Input: part model. Units: mm. Frame: model coordinates. A direction names the side the tool comes from. Give positions to 0.01 mm unless a question says otherwise; leave off trailing zeros. Loops run counter-clockwise (first coordinate to the right, second up) from the corner with the lowest first, then second, coordinate; pieces in that order, holes last. Notation, with made-up numbers: (-16, 36) -> (16, 36) arc R25 ccw to (16, 57) -> close; hole circle Ø3 at (87.25, -6). An arc over 180 degrees is marked (long way). Answer as a JSON object with one key per item and string values.
```python
from build123d import *

# Parameters (mm, degrees)
F0_R     = 12.5
F0_R_2   = 9.5
F0_R_3   = 3.5
F1_DEPTH = 20
F2_DEPTH = 5
F3_R     = 1.5
F4_SIZE  = 0.99999
F5_SIZE  = 1


# Not quite as in the source:
# - a fillet or chamfer is up to 0.001 mm smaller than in the source, because OpenCascade refuses the exact size


with BuildPart() as f1:
    # F0 (on Top) → F1 (new body)
    with BuildSketch(Plane.XY):
        with BuildLine():
            Line((50, 27.5), (-50, 27.5))
            ThreePointArc((-50, 27.5), (-53.5355339059, 26.0355339059), (-55, 22.5))
            Line((-55, 22.5), (-55, -22.5))
            ThreePointArc((-55, -22.5), (-53.5355339059, -26.0355339059), (-50, -27.5))
            Line((-50, -27.5), (50, -27.5))
            ThreePointArc((50, -27.5), (53.5355339059, -26.0355339059), (55, -22.5))
            Line((55, -22.5), (55, 22.5))
            ThreePointArc((55, 22.5), (53.5355339059, 26.0355339059), (50, 27.5))
        make_face()
        with Locations((-37.5, -12)):
            Circle(F0_R, mode=Mode.SUBTRACT)
        with BuildLine():
            ThreePointArc((0, -12), (-12.5, -24.5), (-25, -12))
            ThreePointArc((-25, -12), (-12.5, 0.5), (0, -12))
        make_face(mode=Mode.SUBTRACT)
        with BuildLine():
            ThreePointArc((25, -12), (12.5, -24.5), (0, -12))
            ThreePointArc((0, -12), (12.5, 0.5), (25, -12))
        make_face(mode=Mode.SUBTRACT)
        with BuildLine():
            ThreePointArc((50, -12), (37.5, -24.5), (25, -12))
            ThreePointArc((25, -12), (37.5, 0.5), (50, -12))
        make_face(mode=Mode.SUBTRACT)
        with Locations((-43, 15)):
            Circle(F0_R_2, mode=Mode.SUBTRACT)
        with Locations((-21.5, 15)):
            Circle(F0_R_2, mode=Mode.SUBTRACT)
        with Locations((0, 15)):
            Circle(F0_R_2, mode=Mode.SUBTRACT)
        with Locations((21.5, 15)):
            Circle(F0_R_2, mode=Mode.SUBTRACT)
        with Locations((43, 15)):
            Circle(F0_R_2, mode=Mode.SUBTRACT)
        with BuildLine():
            ThreePointArc((0, -12), (-12.5, 0.5), (-25, -12))
            ThreePointArc((-25, -12), (-12.5, -24.5), (0, -12))
        make_face()
        with Locations((-12.5, -12)):
            Circle(F0_R_3, mode=Mode.SUBTRACT)
        with Locations((-37.5, -12)):
            Circle(F0_R)
        with Locations((-37.5, -12)):
            Circle(F0_R_3, mode=Mode.SUBTRACT)
        with BuildLine():
            ThreePointArc((25, -12), (12.5, 0.5), (0, -12))
            ThreePointArc((0, -12), (12.5, -24.5), (25, -12))
        make_face()
        with Locations((12.5, -12)):
            Circle(F0_R_3, mode=Mode.SUBTRACT)
        with BuildLine():
            ThreePointArc((50, -12), (37.5, 0.5), (25, -12))
            ThreePointArc((25, -12), (37.5, -24.5), (50, -12))
        make_face()
        with Locations((37.5, -12)):
            Circle(F0_R_3, mode=Mode.SUBTRACT)
    extrude(amount=F1_DEPTH)

    # F0 (on Top) → F2 (join)
    with BuildSketch(Plane.XY):
        with Locations((-43, 15)):
            Circle(F0_R_2)
        with Locations((-21.5, 15)):
            Circle(F0_R_2)
        with Locations((0, 15)):
            Circle(F0_R_2)
        with Locations((21.5, 15)):
            Circle(F0_R_2)
        with Locations((43, 15)):
            Circle(F0_R_2)
    extrude(amount=F2_DEPTH)

    # F3
    f3_edges = [f1.edges().sort_by_distance(p)[0] for p in [
        (0, -27.5, 20),
    ]]
    fillet(f3_edges, radius=F3_R)

    # F4 (size 1 in the source; OpenCascade refuses exactly that, so slightly less here)
    f4_edges = [f1.edges().sort_by_distance(p)[0] for p in [
        (-52.5, 15, 20),
        (-31, 15, 20),
        (-9.5, 15, 20),
        (12, 15, 20),
        (33.5, 15, 20),
    ]]
    chamfer(f4_edges, length=F4_SIZE)

    # F5
    f5_edges = [f1.edges().sort_by_distance(p)[0] for p in [
        (-41, -12, 20),
        (-16, -12, 20),
        (9, -12, 20),
        (34, -12, 20),
    ]]
    chamfer(f5_edges, length=F5_SIZE)


solid = f1.part
```
Q1. Section C-C, the plane z = 15.5. Give the number of separate pieces and of enclosed holes in the cut face, then the cut area to 3 significant figures.
Evaluation:
{"separate pieces": "1", "enclosed holes": "9", "area": "4,460 mm2"}
Q2. Access query for faces 4 (the flat face through (-1, -5, 20)), 5 (the cylindrical face through (30.276, 11.361, 11.902)). Directions: +Z, -Z, +X, -X, +Y, -Y. A direction counts if a zero-diameter tool reaches every point of the face in a straight line with its end or side. Return the directions, or none.
Evaluation:
{"face 4": "+Z, +X, -X, +Y, -Y", "face 5": "+Z"}
Q3. Pin query (flat end, axial travel): pin 1 (11.5 mm diameter, centred on x = -43, y = 15, fed in from -Z); pin 2 (8 mm diameter, centred on x = -12.5, y = -12, fed in from +Z); pin 3 (5.5 mm diameter, centred on x = -42.5, y = 14.5, fed in from +Z). Return the tip coordinate at first contact, or that it passes through.
Evaluation:
{"pin 1": "stops at z = 0", "pin 2": "stops at z = 19.5", "pin 3": "stops at z = 5"}
Q4. Section A-A, the plane z = 2.5. Return the cut outline in (x, y), then the cut area to 3 significant figures.
Evaluation:
{"outline": "(-55, -22.5) arc R5 ccw to (-50, -27.5) -> (50, -27.5) arc R5 ccw to (55, -22.5) -> (55, 22.5) arc R5 ccw to (50, 27.5) -> (-50, 27.5) arc R5 ccw to (-55, 22.5) -> close; hole circle Ø7 at (-37.5, -12); hole circle Ø7 at (-12.5, -12); hole circle Ø7 at (12.5, -12); hole circle Ø7 at (37.5, -12)", "area": "5,870 mm2"}
Q5. Ray query, line 1 along X through (y, z) = (14.5, 7); line 2 along Y through (x, z) = (38, 7); line 3 along Y through (x, z) = (-43, 14). Return the intervals inside material, ascending.
Evaluation:
{"line 1": "x = -55 to -52.49, -33.51 to -30.99, -12.01 to -9.49, 9.49 to 12.01, 30.99 to 33.51, 52.49 to 55", "line 2": "y = -27.5 to -15.46, -8.54 to 6.92, 23.08 to 27.5", "line 3": "y = -27.5 to 5.5, 24.5 to 27.5"}
Q6. Section B-B, the plane x = 21.5. Return the cut outline in (y, z), then the cut area to 3 significant figures.
Evaluation:
{"outline": "(-27.5, 0) -> (27.5, 0) -> (27.5, 18.5) arc R1.5 ccw to (26, 20) -> (25.5, 20) -> (24.5, 19) -> (24.5, 5) -> (5.5, 5) -> (5.5, 19) -> (4.5, 20) -> (-26, 20) arc R1.5 ccw to (-27.5, 18.5) -> close", "area": "813 mm2"}
Q7. Draft query along Y for faces 1 (the cylindrical face through (-40.3, -14.1, 9.4)), 2 (the flat face through (-55, 0, 9)), 3 (the cylindrical face through (53.57, 26, 9.12)). Return one class per face: +Y half, -Y half, draft (parallel to the pull), parting line (faces both ways), or undercut.
Evaluation:
{"face 1": "undercut", "face 2": "draft", "face 3": "+Y half"}
